Autodesk Inventor part; units mm, degrees
ref_plane "YZ Plane" through (0, 0, 0) normal (1, 0, 0) x (0, 1, 0)
ref_plane "XZ Plane" through (0, 0, 0) normal (0, 1, 0) x (-1, 0, 0)
ref_plane "XY Plane" through (0, 0, 0) normal (0, 0, 1) x (1, 0, 0)
sketch "Sketch1" plane through (0, 0, 0) normal (0, 0, 1) x (1, 0, 0)
  line L0 (0, 0) -> (101.6, 0)
  line L1 (101.6, 0) -> (101.6, 76.2)
  line L2 (101.6, 76.2) -> (25.4, 76.2)
  line L3 (0, 0) -> (0, 25.4)
  line L4 (0, 25.4) -> (25.4, 76.2)
  circle A0 centre (12.7, 12.7) radius 3.2512
  circle A1 centre (38.1, 12.7) radius 3.2512
  circle A2 centre (63.5, 12.7) radius 3.2512
  circle A3 centre (88.9, 12.7) radius 3.2512
  circle A4 centre (88.9, 38.1) radius 3.2512
  circle A5 centre (63.5, 38.1) radius 3.2512
  circle A6 centre (38.1, 38.1) radius 3.2512
  circle A7 centre (88.9, 63.5) radius 3.2512
  circle A8 centre (63.5, 63.5) radius 3.2512
  circle A9 centre (38.1, 63.5) radius 3.2512
  dimension "d0" = 101.6
  dimension "d1" = 76.2
  dimension "d2" = 76.2
  dimension "d3" = 25.4
  dimension "d4" = 6.5024
  dimension "d5" = 12.7
  dimension "d6" = 12.7
  dimension "d9" = 25.4
  dimension "d16" = 25.4
extrude "Extrusion1" add sketch "Sketch1" along normal blind 6.35
properties part number "3x1 L PLate"
The model under review builds one solid part; all positions refer to its coordinate system, in mm. Round coordinates to 2 decimals unless told otherwise and drop trailing zeros. Write each loop counter-clockwise with the first axis right and the second up, starting at its lowest first coordinate (ties: lowest second). Pieces come first, ordered by that corner, then holes. Notation, with made-up numbers: (30.25, 44) -> (48.25, 44) arc R24 ccw to (48.25, 83) -> close; hole circle Ø6 at (-31.75, 46). An arc over 180 degrees is marked (long way). Answer as a JSON object with one key per item and string values.
1. The part is to be moulded in two halves that separate along X. For faces 1 (the face through (0, 13, 3)), 2 (the face through (101.6, 38, 3)), 3 (the face through (60.25, 12.56, 3.13)), 4 (the face through (50, 39, 6.35)), say which applies: pulls with the +X half, pulls with the -X half, needs draft (parallel to the pull), parting line crosses it, or undercut.
Results found:
{"face 1": "pulls with the -X half", "face 2": "pulls with the +X half", "face 3": "undercut", "face 4": "needs draft"}
2. We need section C-C on x = 88.9. State the section outline as (y, z) points, and give its area (3 significant figures).
Results found:
{"outline": "(0, 0) -> (9.45, 0) -> (9.45, 6.35) -> (0, 6.35) -> close; (15.95, 0) -> (34.85, 0) -> (34.85, 6.35) -> (15.95, 6.35) -> close; (41.35, 0) -> (60.25, 0) -> (60.25, 6.35) -> (41.35, 6.35) -> close; (66.75, 0) -> (76.2, 0) -> (76.2, 6.35) -> (66.75, 6.35) -> close", "area": "360 mm^2"}
3. Clearance check with a flat-ended pin moving along its axis: pin 1 (7.5 mm diameter, centred on x = 63.5, y = 63.5, fed in from +Z). State where the tip first meets the part, or that it passes through.
Results found:
{"pin 1": "stops at z = 6.35"}
4. We need section D-D on y = 12.7. State the section outline as (x, z) points, and give its area (3 significant figures).
Results found:
{"outline": "(0, 0) -> (9.45, 0) -> (9.45, 6.35) -> (0, 6.35) -> close; (15.95, 0) -> (34.85, 0) -> (34.85, 6.35) -> (15.95, 6.35) -> close; (41.35, 0) -> (60.25, 0) -> (60.25, 6.35) -> (41.35, 6.35) -> close; (66.75, 0) -> (85.65, 0) -> (85.65, 6.35) -> (66.75, 6.35) -> close; (92.15, 0) -> (101.6, 0) -> (101.6, 6.35) -> (92.15, 6.35) -> close", "area": "480 mm^2"}
5. We need section A-A on y = 38.1. State the section outline as (x, z) points, and give its area (3 significant figures).
Results found:
{"outline": "(6.35, 0) -> (34.85, 0) -> (34.85, 6.35) -> (6.35, 6.35) -> close; (41.35, 0) -> (60.25, 0) -> (60.25, 6.35) -> (41.35, 6.35) -> close; (66.75, 0) -> (85.65, 0) -> (85.65, 6.35) -> (66.75, 6.35) -> close; (92.15, 0) -> (101.6, 0) -> (101.6, 6.35) -> (92.15, 6.35) -> close", "area": "481 mm^2"}
6. To check wall thickness, follow line 1 along Y through (x, z) = (38.1, 2.5); line 2 along X through (y, z) = (40.5, 2.75). State the ranges of each line that lie inside material, in increasing order.
Results found:
{"line 1": "y = 0 to 9.45, 15.95 to 34.85, 41.35 to 60.25, 66.75 to 76.2", "line 2": "x = 7.55 to 35.91, 40.29 to 61.31, 65.69 to 86.71, 91.09 to 101.6"}
7. We need section B-B on x = 12.7. State the section outline as (y, z) points.
Results found:
{"outline": "(0, 0) -> (9.45, 0) -> (9.45, 6.35) -> (0, 6.35) -> close; (15.95, 0) -> (50.8, 0) -> (50.8, 6.35) -> (15.95, 6.35) -> close"}
